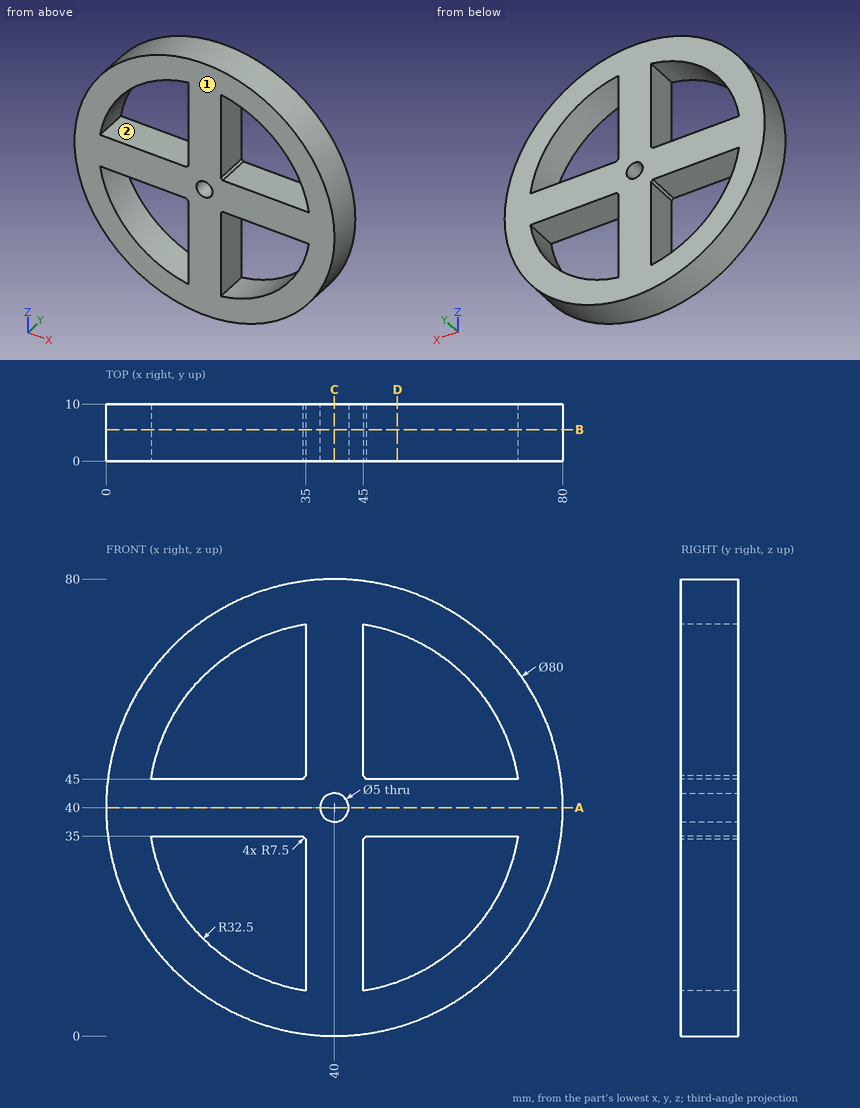
Can you work these out from the drawing? Everything is in mm from the part's minimum corner. A direction names the side the tool comes from. Coordinates: 2 decimals unless noted, no trailing zeros. Order: outer loops, then holes, each group sorted by start corner. A loop starts at its lowest first (then second) coordinate and runs counter-clockwise, first axis right, second up. Notation, with made-up numbers: (38, 38.5) -> (91, 38.5) arc R16 ccw to (91, 52.5) -> close; hole circle Ø2 at (60, 73.25). An arc over 180 degrees is marked (long way). Use one line per item in the form item = value.
Q1. Imagine slicing it at A-A, the plane z = 40. List the corners of the cut face in (x, y) for me.
From the geometry:
outline = (0, 0) -> (37.5, 0) -> (37.5, 10) -> (0, 10) -> close; (42.5, 0) -> (80, 0) -> (80, 10) -> (42.5, 10) -> close
Q2. Which directions (+Z, -Z, +X, -X, +Y, -Y) give clear straight access to the entire face, cutting with the end or side of a thin tool? Please do the marked faces 1 and 2.
From the geometry:
face_1 = +Z, -Z, +X, -X, -Y
face_2 = +Y, -Y
Q3. Imagine slicing it at C-C, the plane x = 40. List the corners of the cut face in (y, z) for me.
From the geometry:
outline = (0, 0) -> (10, 0) -> (10, 37.5) -> (0, 37.5) -> close; (0, 42.5) -> (10, 42.5) -> (10, 80) -> (0, 80) -> close
Q4. Imagine slicing it at D-D, the plane x = 51. List the corners of the cut face in (y, z) for me, then the cut area to 4 significant figures.
From the geometry:
outline = (0, 1.54) -> (10, 1.54) -> (10, 9.42) -> (0, 9.42) -> close; (0, 35) -> (10, 35) -> (10, 45) -> (0, 45) -> close; (0, 70.58) -> (10, 70.58) -> (10, 78.46) -> (0, 78.46) -> close
area = 257.5 mm²
Q5. I need wall thicknesses on L1, parallel to X at y = 5, z = 30; L2, parallel to Z at x = 40, y = 6.5; L3, parallel to Z at x = 46, y = 9.75. Which ranges of each line are inside material? Lowest first, please.
From the geometry:
L1 = 1.27 to 9.08, 35 to 45, 70.92 to 78.73
L2 = 0 to 37.5, 42.5 to 80
L3 = 0.45 to 8.06, 35 to 45, 71.94 to 79.55
Q6. Imagine slicing it at B-B, the plane y = 5.5. List the corners of the cut face in (x, z) for me.
From the geometry:
outline = circle Ø80 at (40, 40); hole (7.89, 35) arc R32.5 ccw to (35, 7.89) -> (35, 34.41) arc R7.5 cw to (34.41, 35) -> close; hole (7.89, 45) -> (34.41, 45) arc R7.5 cw to (35, 45.59) -> (35, 72.11) arc R32.5 ccw to start; hole circle Ø5 at (40, 40); hole (45, 7.89) arc R32.5 ccw to (72.11, 35) -> (45.59, 35) arc R7.5 cw to (45, 34.41) -> close; hole (45, 45.59) arc R7.5 cw to (45.59, 45) -> (72.11, 45) arc R32.5 ccw to (45, 72.11) -> close
Q7. Will these pins go through, and if not, where does the flat tip stop? P1, Ø3, axis at x = 33, z = 49, coming from the +Y side; P2, Ø3, axis at y = 4.5, z = 52, coming from the +X side; P3, Ø3, axis at x = 24.5, y = 6.5, coming from the -Z side; P4, Ø3, axis at x = 18.5, y = 4, coming from the +Z side.
From the geometry:
P1 = through
P2 = 78.6
P3 = 2.53
P4 = 74.64
